from build123d import *

# Parameters (mm, degrees)
BOSS_EXTRUDE1_DEPTH                             = 2.5
CSK_FOR_M2_FLAT_HEAD_MACHINE_SCREW1_D           = 2.4
CSK_FOR_M2_FLAT_HEAD_MACHINE_SCREW1_CSINK_D     = 4.4
CSK_FOR_M2_FLAT_HEAD_MACHINE_SCREW1_CSINK_ANGLE = 90
SKETCH6_R                                       = 1.5
BOSS_EXTRUDE2_DEPTH                             = 10.5
SKETCH7_R                                       = 9
CUT_EXTRUDE1_DEPTH                              = 10.5
SKETCH8_R                                       = 2
BOSS_EXTRUDE3_DEPTH                             = 2.5
BOSS_EXTRUDE4_DEPTH                             = 2
FILLET1_R                                       = 1
FILLET2_R                                       = 0.5


with BuildPart() as part:
    # Sketch1 → Boss-Extrude1 (new body)
    with BuildSketch(Plane(origin=(0, 0, 0), x_dir=(1, 0, 0), z_dir=(0, 1, 0))):
        Polygon((10, 0), (190, 0), (200, -10), (200, -90), (190, -100), (10, -100), (0, -90), (0, -10), align=None)
    extrude(amount=BOSS_EXTRUDE1_DEPTH)

    # CSK for M2 Flat Head Machine Screw1 (through all)
    with Locations(Plane(origin=(0, 0, 0), x_dir=(-1, 0, 0), z_dir=(0, -1, 0))):
        with Locations((-190, -10), (-190, -90), (-10, -10), (-10, -90)):
            CounterSinkHole(CSK_FOR_M2_FLAT_HEAD_MACHINE_SCREW1_D / 2, CSK_FOR_M2_FLAT_HEAD_MACHINE_SCREW1_CSINK_D / 2, counter_sink_angle=CSK_FOR_M2_FLAT_HEAD_MACHINE_SCREW1_CSINK_ANGLE)

    # Sketch6 → Boss-Extrude2 (add)
    with BuildSketch(Plane(origin=(0, 2.5, 0), x_dir=(1, 0, 0), z_dir=(0, 1, 0))):
        with Locations(Location((11.75, -29.5, 0), (0, 0, 90))):
            Circle(SKETCH6_R)
        with Locations(Location((11.75, -70.5, 0), (0, 0, 90))):
            Circle(SKETCH6_R)
        with Locations(Location((28.25, -70.5, 0), (0, 0, 90))):
            Circle(SKETCH6_R)
        with Locations(Location((28.25, -29.5, 0), (0, 0, 90))):
            Circle(SKETCH6_R)
    extrude(amount=BOSS_EXTRUDE2_DEPTH)

    # Sketch7 → Cut-Extrude1 (cut)
    with BuildSketch(Plane(origin=(0, 2.5, 0), x_dir=(1, 0, 0), z_dir=(0, 1, 0))):
        with Locations(Location((20, -37, 0), (0, 0, 270))):
            Circle(SKETCH7_R)
        with Locations(Location((20, -63, 0), (0, 0, 270))):
            Circle(SKETCH7_R)
    extrude(amount=-CUT_EXTRUDE1_DEPTH, mode=Mode.SUBTRACT)

    # Sketch8 → Boss-Extrude3 (add)
    with BuildSketch(Plane(origin=(0, 2.5, 0), x_dir=(1, 0, 0), z_dir=(0, 1, 0))):
        with Locations(Location((121, -25.5, 0), (0, 0, 90))):
            Circle(SKETCH8_R)
        with Locations(Location((121, -74.5, 0), (0, 0, 90))):
            Circle(SKETCH8_R)
        with Locations(Location((179, -74.5, 0), (0, 0, 90))):
            Circle(SKETCH8_R)
        with Locations(Location((179, -25.5, 0), (0, 0, 90))):
            Circle(SKETCH8_R)
    extrude(amount=BOSS_EXTRUDE3_DEPTH)

    # Sketch9 → Boss-Extrude4 (add)
    with BuildSketch(Plane(origin=(0, 2.5, 0), x_dir=(1, 0, 0), z_dir=(0, 1, 0))):
        Polygon((170.333333333, -96), (173, -100), (170.333333333, -100), align=None)
        Polygon((196, -70.333333333), (200, -73), (200, -70.333333333), align=None)
        Polygon((0, -70.333333333), (0, -73), (4, -70.333333333), align=None)
        Polygon((29.666666667, -100), (27, -100), (29.666666667, -96), align=None)
        Polygon((29.666666667, -4), (27, 0), (29.666666667, 0), align=None)
        Polygon((4, -29.666666667), (0, -27), (0, -29.666666667), align=None)
        Polygon((200, -29.666666667), (200, -27), (196, -29.666666667), align=None)
        Polygon((170.333333333, 0), (173, 0), (170.333333333, -4), align=None)
    extrude(amount=BOSS_EXTRUDE4_DEPTH)

    # Fillet1
    fillet1_edges = [part.edges().sort_by_distance(p)[0] for p in [
        (200, 2.5, 50),
        (100, 0, 0),
        (200, 2.5, 18.5),
        (100, 2.5, 0),
        (18.5, 2.5, 0),
        (0, 2.5, 50),
        (0, 2.5, 81.5),
        (100, 2.5, 100),
        (181.5, 2.5, 100),
        (195, 0, 5),
        (200, 0, 50),
        (195, 0, 95),
        (195, 2.5, 5),
        (190, 1.25, 100),
        (10, 1.25, 100),
        (0, 1.25, 90),
        (0, 1.25, 10),
        (10, 1.25, 0),
        (190, 1.25, 0),
        (200, 1.25, 10),
        (200, 1.25, 90),
        (181.5, 2.5, 0),
        (5, 2.5, 5),
        (0, 2.5, 18.5),
        (5, 2.5, 95),
        (18.5, 2.5, 100),
        (195, 2.5, 95),
        (100, 0, 100),
        (200, 2.5, 81.5),
        (5, 0, 95),
        (0, 0, 50),
        (5, 0, 5),
    ]]
    fillet(fillet1_edges, radius=FILLET1_R)

    # Fillet2
    fillet2_edges = [part.edges().sort_by_distance(p)[0] for p in [
        (29.666666667, 3.5, 96),
        (29.666666667, 3, 100),
        (27, 3, 100),
        (4, 3.5, 70.333333333),
        (0, 3, 73),
        (0, 3, 70.333333333),
        (4, 3.5, 29.666666667),
        (0, 3, 29.666666667),
        (0, 3, 27),
        (29.666666667, 3, 0),
        (27, 3, 0),
        (29.666666667, 3.5, 4),
        (173, 3, 0),
        (170.333333333, 3, 0),
        (170.333333333, 3.5, 4),
        (196, 3.5, 29.666666667),
        (200, 3, 27),
        (200, 3, 29.666666667),
        (196, 3.5, 70.333333333),
        (200, 3, 70.333333333),
        (200, 3, 73),
        (170.333333333, 3.5, 96),
        (170.333333333, 3, 100),
        (173, 3, 100),
    ]]
    fillet(fillet2_edges, radius=FILLET2_R)


solid = part.part
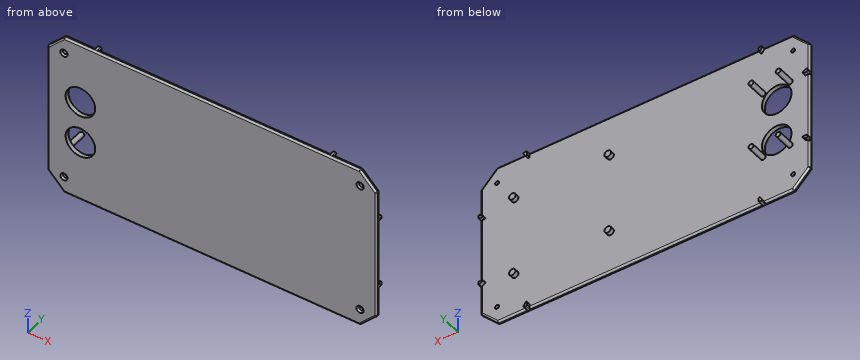
Work out the finished part from the listing and answer in its coordinate system (mm). Give positions to 0.01 mm unless a question says otherwise; leave off trailing zeros. Loops run counter-clockwise (first coordinate to the right, second up) from the corner with the lowest first, then second, coordinate; pieces in that order, holes last. Notation, with made-up numbers: M 77,-23.75 L 109,-23.75 A15 ccw 109,-18.75 Z; hole C 22.25,-0.5 d4. An arc over 180 degrees is marked long. Use CSV: the item, a comma, the result in double quotes.
1) Consider L1, parallel to X at y = 8.75, z = 29.5; L2, parallel to Z at x = 10, y = 2.05; L3, parallel to Z at x = 190, y = 1.7. Determine where each line is inside the solid, lowest interval first.
Answer:
L1,"10.25 to 13.25, 26.75 to 29.75"
L2,"0.27 to 8.8, 11.2 to 88.8, 91.2 to 99.73"
L3,"0.11 to 8.8, 11.2 to 88.8, 91.2 to 99.89"
2) Find section D-D on z = 74.5. Write down the section's boundary in (x, y), plus the area to 3 significant figures.
Answer:
outline,"M 0,1 A1 ccw 1,0 L 199,0 A1 ccw 200,1 L 200,1.5 A1 ccw 199,2.5 L 181,2.5 L 181,5 L 177,5 L 177,2.5 L 123,2.5 L 123,5 L 119,5 L 119,2.5 L 1,2.5 A1 ccw 0,1.5 Z"
area,"519 mm^2"
3) Given P1, Ø0.7, axis at x = 198.5, z = 28.5, coming from the +Y side; P2, Ø12, axis at x = 148.5, z = 61, coming from the +Y side; P3, Ø3, axis at x = 10, z = 90, coming from the -Y side; P4, Ø8, axis at x = 49.5, z = 86.5, coming from the -Y side, each flat-ended and moving along its own axis, determine where each tip first touches the part or whether it passes through.
Answer:
P1,"y = 4.5"
P2,"y = 2.5"
P3,"y = 0.7"
P4,"y = 0"
4) Find section B-B on z = 37. Write down the section's boundary in (x, y), plus the area to 3 significant figures.
Answer:
outline,"M 0,1 A1 ccw 1,0 L 11,0 L 11,2.5 L 1,2.5 A1 ccw 0,1.5 Z; M 29,0 L 199,0 A1 ccw 200,1 L 200,1.5 A1 ccw 199,2.5 L 29,2.5 Z"
area,"454 mm^2"
5) Find section A-A on x = 20. Write down the section's boundary in (y, z).
Answer:
outline,"M 0,1 A1 ccw 1,0 L 1.5,0 A1 ccw 2.5,1 L 2.5,28 L 0,28 Z; M 0,46 L 2.5,46 L 2.5,54 L 0,54 Z; M 0,72 L 2.5,72 L 2.5,99 A1 ccw 1.5,100 L 1,100 A1 ccw 0,99 Z"
6) Find section C-C on y = 7.75. Write down the section's boundary in (x, z).
Answer:
outline,"C 11.75,29.5 d3; C 11.75,70.5 d3; C 28.25,29.5 d3; C 28.25,70.5 d3"
